Design review of the part shown in the three views and the two pictorial views. Dimensions are in mm from the part's minimum x, y and z. Coordinates: 2 decimals unless noted, no trailing zeros. Loops run counter-clockwise (first coordinate to the right, second up) from the corner with the lowest first, then second, coordinate; pieces in that order, holes last. Notation, with made-up numbers: (-29.75, -3.75) -> (28.25, -3.75) arc R32 ccw to (28.25, 32.25) -> close; hole circle Ø5 at (-6, 6). An arc over 180 degrees is marked (long way). Answer in a Markdown table with one row per item.
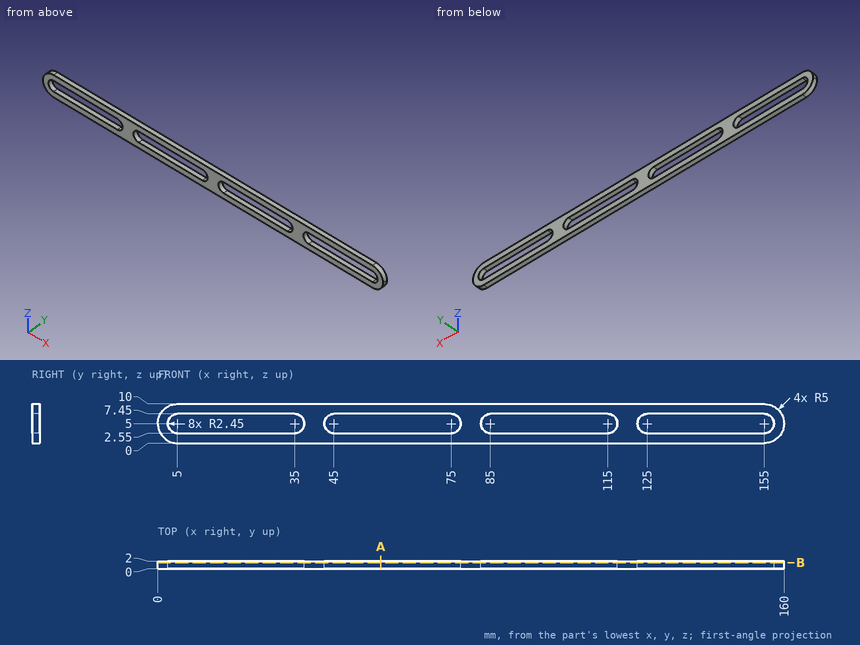
Item 1: For L1, parallel to Z at x = 109, y = 1.2; L2, parallel to X at y = 0.8, z = 4.5 (1 decimal), list the stretches that pass through material, from the lowest coordinate up.
Worked answers:
| item | result |
|---|---|
| L1 | 0 to 2.55, 7.45 to 10 |
| L2 | 0 to 2.6, 37.4 to 42.6, 77.4 to 82.6, 117.4 to 122.6, 157.4 to 160 |
Item 2: Take a section at A-A, the plane x = 57. State the section outline as (y, z) points, and give its area (3 significant figures).
Worked answers:
| item | result |
|---|---|
| outline | (0, 0) -> (2, 0) -> (2, 2.55) -> (0, 2.55) -> close; (0, 7.45) -> (2, 7.45) -> (2, 10) -> (0, 10) -> close |
| area | 10.2 mm² |
Item 3: Take a section at B-B, the plane y = 1.6. Count the separate pieces of the cut face and the enclosed holes in it, and give its area (3 significant figures).
Worked answers:
| item | result |
|---|---|
| separate pieces | 1 |
| enclosed holes | 4 |
| area | 915 mm² |
